Verification items for the finished model (mm, model axes). Give positions to 0.01 mm unless a question says otherwise; leave off trailing zeros. Order: outer loops, then holes, each group sorted by start corner. A loop starts at its lowest first (then second) coordinate and runs counter-clockwise, first axis right, second up. Notation, with made-up numbers: (69, 36) -> (97, 36) arc R14 cw to (97, 62) -> close; hole circle Ø11 at (38, -23.5). An arc over 180 degrees is marked (long way). Return JSON: item names as keys, results as strings. Group by question number.
(1) Cross-section at B-B on x = 737. Enter the section's corners in (y, z) (3 decimals).
(2) Cross-section at C-C on z = 10.5. Enter the section's corners in (x, y) (3 decimals).
(3) Thickness scan on line 1 along X through (y, z) = (-266.5, 21) (3 decimals); line 2 along Y through (x, z) = (699, 21) (3 decimals); line 3 along Y through (x, z) = (545.5, 2.5). Record the ranges inside material, lowest first.
(4) Cross-section at A-A on y = -758. Enter the section's corners in (x, z) (3 decimals), then the cut area to 3 significant figures.
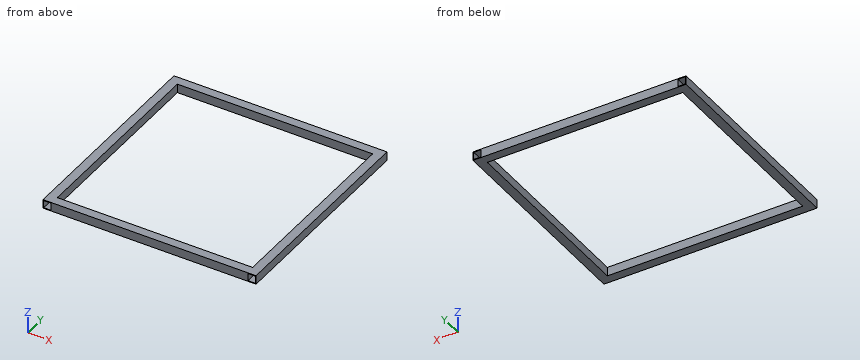
from build123d import *

# Parameters (mm, degrees)
F0_W     = 38.1
F0_H     = 38.1
F0_W_2   = 31.75
F0_H_2   = 31.75
F1_DEPTH = 914.4
F2_W     = 38.1
F2_H     = 38.1
F2_W_2   = 31.75
F2_H_2   = 31.75
F3_DEPTH = 838.2


with BuildPart() as f1:
    # F0 (on Front) → F1 (new body)
    with BuildSketch(Plane.XZ):
        with Locations((19.05, 19.05)):
            Rectangle(F0_W, F0_H)
        with Locations((19.05, 19.05)):
            Rectangle(F0_W_2, F0_H_2, mode=Mode.SUBTRACT)
        with Locations((895.35, 19.05)):
            Rectangle(F0_W, F0_H)
        with Locations((895.35, 19.05)):
            Rectangle(F0_W_2, F0_H_2, mode=Mode.SUBTRACT)
    extrude(amount=F1_DEPTH)

    # F2 (on face) → F3 (join)
    with BuildSketch(Plane.YZ.offset(38.1)):
        with Locations((-895.35, 19.05)):
            Rectangle(F2_W, F2_H)
        with Locations((-895.35, 19.05)):
            Rectangle(F2_W_2, F2_H_2, mode=Mode.SUBTRACT)
        with Locations((-19.05, 19.05)):
            Rectangle(F2_W, F2_H)
        with Locations((-19.05, 19.05)):
            Rectangle(F2_W_2, F2_H_2, mode=Mode.SUBTRACT)
    extrude(amount=F3_DEPTH)


solid = f1.part
Verdict:
{
 "1": {"outline": "(-914.4, 0) -> (-876.3, 0) -> (-876.3, 38.1) -> (-914.4, 38.1) -> close; (-38.1, 0) -> (0, 0) -> (0, 38.1) -> (-38.1, 38.1) -> close; hole (-911.225, 3.175) -> (-879.475, 3.175) -> (-879.475, 34.925) -> (-911.225, 34.925) -> close; hole (-34.925, 3.175) -> (-3.175, 3.175) -> (-3.175, 34.925) -> (-34.925, 34.925) -> close"},
 "2": {"outline": "(0, -914.4) -> (3.175, -914.4) -> (3.175, 0) -> (0, 0) -> close; (34.925, -914.4) -> (879.475, -914.4) -> (879.475, 0) -> (34.925, 0) -> close; (911.225, -914.4) -> (914.4, -914.4) -> (914.4, 0) -> (911.225, 0) -> close; hole (38.1, -911.225) -> (876.3, -911.225) -> (876.3, -879.475) -> (38.1, -879.475) -> close; hole (38.1, -876.3) -> (876.3, -876.3) -> (876.3, -38.1) -> (38.1, -38.1) -> close; hole (38.1, -34.925) -> (876.3, -34.925) -> (876.3, -3.175) -> (38.1, -3.175) -> close"},
 "3": {"line 1": "0 to 3.175, 34.925 to 38.1, 876.3 to 879.475, 911.225 to 914.4", "line 2": "-914.4 to -911.225, -879.475 to -876.3, -38.1 to -34.925, -3.175 to 0", "line 3": "-914.4 to -876.3, -38.1 to 0"},
 "4": {"outline": "(0, 0) -> (38.1, 0) -> (38.1, 38.1) -> (0, 38.1) -> close; (876.3, 0) -> (914.4, 0) -> (914.4, 38.1) -> (876.3, 38.1) -> close; hole (3.175, 3.175) -> (34.925, 3.175) -> (34.925, 34.925) -> (3.175, 34.925) -> close; hole (879.475, 3.175) -> (911.225, 3.175) -> (911.225, 34.925) -> (879.475, 34.925) -> close", "area": "887 mm²"}
}
